Autodesk Inventor part; units mm, degrees
ref_plane "YZ Plane" through (0, 0, 0) normal (1, 0, 0) x (0, 1, 0)
ref_plane "XZ Plane" through (0, 0, 0) normal (0, 1, 0) x (-1, 0, 0)
ref_plane "XY Plane" through (0, 0, 0) normal (0, 0, 1) x (1, 0, 0)
sketch "Sketch1" plane through (0, 0, 0) normal (0, 1, 0) x (-1, 0, 0)
  line L0 (0, 0) -> (90, 0)
  line L1 (90, 0) -> (90, -52)
  line L2 (90, -60) -> (0, -60)
  line L3 (0, -60) -> (0, 0)
  line L4 (0, 0) -> (90, 0)
  line L5 (90, 0) -> (90, -8)
  line L6 (90, -8) -> (0, -8)
  line L7 (0, -8) -> (0, 0)
  line L8 (90, -60) -> (0, -60)
  line L9 (0, -60) -> (0, -52)
  line L10 (0, -52) -> (90, -52)
  line L11 (90, -52) -> (90, -60)
  line L12 (0, -8) -> (90, -8)
  line L13 (90, -8) -> (90, -12)
  line L14 (90, -12) -> (0, -12)
  line L15 (0, -12) -> (0, -8)
  line L16 (90, -52) -> (0, -52)
  line L17 (0, -52) -> (0, -48)
  line L18 (0, -48) -> (90, -48)
  line L19 (90, -48) -> (90, -52)
  line L20 (90, 0) -> (64, 0)
  line L21 (64, 0) -> (64, -8)
  line L22 (64, -8) -> (90, -8)
  line L23 (90, -8) -> (90, 0)
  line L24 (64, -8) -> (57, -8)
  line L25 (57, -8) -> (57, 0)
  line L26 (57, 0) -> (64, 0)
  line L27 (64, 0) -> (64, -8)
  line L28 (57, 0) -> (24, 0)
  line L29 (24, 0) -> (24, -8)
  line L30 (24, -8) -> (57, -8)
  line L31 (57, -8) -> (57, 0)
  line L32 (24, -8) -> (17, -8)
  line L33 (17, -8) -> (17, 0)
  line L34 (17, 0) -> (24, 0)
  line L35 (24, 0) -> (24, -8)
  line L36 (57, 0) -> (50, 0)
  line L37 (50, 0) -> (50, -8)
  line L38 (50, -8) -> (57, -8)
  line L39 (57, -8) -> (57, 0)
  line L40 (64, -52) -> (57, -52)
  line L41 (57, -52) -> (57, -60)
  line L42 (57, -60) -> (64, -60)
  line L43 (64, -60) -> (64, -52)
  line L44 (24, -52) -> (17, -52)
  line L45 (17, -52) -> (17, -60)
  line L46 (17, -60) -> (24, -60)
  line L47 (24, -60) -> (24, -52)
  dimension "d0" = 90
  dimension "d1" = 60
  dimension "d49" = 8
  dimension "d50" = 8
extrude "Extrusion1" add sketch "Sketch1" along normal blind 4 contours L14 L1 L18 L3
extrude "Extrusion2" add sketch "Sketch1" along normal blind 40 contours L0 L29 L6 L33 | L6 L1 L14 L3 | L0 L25 L6 L37 | L18 L1 L10 L3 | L0 L21 L6 L25 | L10 L47 L2 L45 | L43 L2 L41 L10
sketch "Sketch2" plane through (0, 40, 0) normal (0, 1, 0) x (1, 0, 0)
  line L0 (-64, 60) -> (-64, 52)
  line L1 (-57, 52) -> (-57, 60)
  circle A0 centre (-60.5, 55.5) radius 1.6
  line L2 (-24, 60) -> (-24, 52)
  circle A1 centre (-20.5, 56) radius 1.6
  line L3 (-90, 8) -> (-64, 8)
  circle A2 centre (-60.5, 4) radius 1.6
  line L4 (-17, 0) -> (-17, 8)
  line L5 (-24, 0) -> (-17, 0)
  circle A3 centre (-20.5, 4) radius 1.6
  point P0 (0, 0)
  point P1 (-17, 52)
  dimension "d6" = 3.2
  dimension "d7" = 3.2
  dimension "d9" = 3.2
  dimension "d10" = 3.2
extrude "Extrusion3" cut sketch "Sketch2" against normal blind 100
sketch "Sketch3" plane through (-64, 0, 0) normal (0, 0, 1) x (1, 0, 0)
  line L0 (0, 0) -> (14, 0)
  line L1 (7, 0) -> (7, 40)
  line L2 (7, 0) -> (7, 40)
  line L3 (0, 40) -> (14, 40)
  circle A0 centre (10.5, 20) radius 1
  circle A1 centre (10.5, 33) radius 1
  circle A2 centre (10.5, 7) radius 1
  point P0 (64, 0)
  dimension "d13" = 2
extrude "Extrusion4" cut sketch "Sketch3" against normal blind 30
sketch "Sketch4" plane through (0, 4, 0) normal (0, 1, 0) x (1, 0, 0)
  line L0 (0, 12) -> (-90, 12)
  line L1 (0, 48) -> (-90, 48)
  line L2 (-90, 12) -> (-86.8, 12)
  line L3 (-86.8, 12) -> (-86.8, 48)
  line L4 (-86.8, 48) -> (-90, 48)
  line L5 (-90, 48) -> (-90, 12)
  line L6 (0, 12) -> (-5, 12)
  line L7 (-5, 12) -> (-5, 48)
  line L8 (-5, 48) -> (0, 48)
  line L9 (0, 48) -> (0, 12)
  line L10 (-17, 12) -> (-10, 12)
  line L11 (-10, 12) -> (-10, 15)
  line L12 (-10, 15) -> (-17, 15)
  line L13 (-17, 15) -> (-17, 12)
  line L14 (-17, 48) -> (-10, 48)
  line L15 (-10, 48) -> (-10, 45)
  line L16 (-10, 45) -> (-17, 45)
  line L17 (-17, 45) -> (-17, 48)
  line L18 (-17, 15) -> (-10, 15)
  line L19 (-10, 21) -> (-17, 21)
  line L20 (-17, 21) -> (-10, 21)
  line L21 (-10, 21) -> (-10, 24)
  line L22 (-10, 24) -> (-17, 24)
  line L23 (-17, 24) -> (-17, 21)
  line L24 (-17, 45) -> (-10, 45)
  line L25 (-10, 39) -> (-17, 39)
  line L26 (-17, 39) -> (-10, 39)
  line L27 (-10, 39) -> (-10, 36)
  line L28 (-10, 36) -> (-17, 36)
  line L29 (-17, 36) -> (-17, 39)
  line L30 (-64, 12) -> (-71, 12)
  line L31 (-71, 12) -> (-71, 15)
  line L32 (-71, 15) -> (-64, 15)
  line L33 (-64, 15) -> (-64, 12)
  line L34 (-64, 21) -> (-71, 21)
  line L35 (-71, 21) -> (-71, 24)
  line L36 (-71, 24) -> (-64, 24)
  line L37 (-64, 24) -> (-64, 21)
  line L38 (-64, 36) -> (-71, 36)
  line L39 (-71, 36) -> (-71, 39)
  line L40 (-71, 39) -> (-64, 39)
  line L41 (-64, 39) -> (-64, 36)
  line L42 (-64, 48) -> (-71, 48)
  line L43 (-71, 48) -> (-71, 45)
  line L44 (-71, 45) -> (-64, 45)
  line L45 (-64, 45) -> (-64, 48)
  line L46 (-10, 48) -> (-17, 48)
  line L47 (-10, 12) -> (-17, 12)
  point P0 (0, 0)
  dimension "d16" = 3.2
extrude "Extrusion5" add sketch "Sketch4" along normal blind 36 contours L0 L7 L1 L9
extrude "Extrusion6" add sketch "Sketch4" along normal blind 36 contours L0 L13 L12 L11 | L15 L16 L17 L1 | L0 L31 L32 L33 | L45 L44 L43 L1
extrude "Extrusion7" add sketch "Sketch4" along normal blind 1 contours L19 L23 L22 L21 | L27 L28 L29 L25 | L34 L35 L36 L37 | L38 L39 L40 L41
sketch "Sketch5" plane through (-5, 4, -48) normal (-1, 0, 0) x (0, 0, 1)
  line L0 (0, 36) -> (36, 36)
  circle A0 centre (18, 22) radius 6
  point P0 (48, -4)
extrude "Extrusion8" cut sketch "Sketch5" against normal blind 20
sketch "Sketch6" plane through (-90, 0, -8) normal (-1, 0, 0) x (0, 0, 1)
  line L0 (0, 0) -> (-44, 0)
  line L1 (-40, 4) -> (-40, 40)
  arc A0 (-28, 12) -> (-16, 12) centre (-22, 20) ccw
  line L2 (-37, 4) -> (-37, 40)
  line L3 (-4, 12) -> (-16, 12)
  line L4 (-28, 12) -> (-37, 12)
  line L5 (-7, 4) -> (-4, 4)
  line L6 (-4, 4) -> (-4, 12)
  line L7 (-4, 40) -> (-4, 4)
  line L8 (-40, 4) -> (-4, 4)
  line L9 (-37, 12) -> (-40, 12)
  line L10 (-40, 12) -> (-40, 4)
  point P0 (8, 0)
  dimension "d30" = 20
extrude "Extrusion9" add sketch "Sketch6" against normal blind 4
sketch "Sketch8" plane through (0, 0, 0) normal (0, -1, 0) x (1, 0, 0)
  line L0 (-64, -52) -> (-90, -52)
  line L1 (-86, -52) -> (-76, -52)
  line L2 (-76, -52) -> (-76, -56)
  line L3 (-76, -56) -> (-86, -56)
  line L4 (-86, -56) -> (-86, -52)
  line L5 (-85, -52) -> (-77, -52)
  line L6 (-77, -52) -> (-77, -55)
  line L7 (-77, -55) -> (-85, -55)
  line L8 (-85, -55) -> (-85, -52)
  line L9 (-85, -55) -> (-77, -55)
  line L10 (-77, -55) -> (-77, -46.5727)
  line L11 (-77, -46.5727) -> (-85, -46.5727)
  line L12 (-85, -46.5727) -> (-85, -55)
  point P0 (0, 0)
extrude "Extrusion14" add sketch "Sketch8" against normal blind 15 contours L2 L3 L4 L0 L8 L7 L6 | L6 L7 L8 L0
extrude "Extrusion15" cut sketch "Sketch8" against normal blind 15 contours L6 L7 L8 L0 | L0 L12 L11 L10
sketch "Sketch9" plane through (0, 0, -52) normal (0, 0, -1) x (-1, 0, 0)
  line L0 (0, 0) -> (0, 40)
  line L1 (0, 0) -> (36, 0)
  line L2 (36, 0) -> (36, 11.5)
  line L3 (36, 11.5) -> (0, 11.5)
  line L4 (0, 11.5) -> (0, 0)
  circle A0 centre (36, 11.5) radius 1
  dimension "d45" = 11.5
  dimension "d46" = 2
extrude "Extrusion16" cut sketch "Sketch9" against normal blind 10 contours A0 L2 L3 | L3 L2 A0
sketch "Sketch10" plane through (-90, 0, -8) normal (-1, 0, 0) x (0, 0, 1)
  line L0 (-44, 0) -> (-52, 0)
  line L1 (-44, 0) -> (-44, 7)
  line L2 (-44, 0) -> (-44, 40)
  circle A0 centre (-33, 7) radius 1.2
  line L3 (0, 0) -> (0, 40)
  line L4 (0, 7) -> (11, 7) construction
  circle A1 centre (-11, 7) radius 1.2
  point P0 (8, 0)
  dimension "d51" = 2.4
  dimension "d54" = 2.4
properties part number "_3DPrint"
The listing builds one solid part. Answer for the finished solid, in the listing's coordinates (mm). A direction names the side the tool comes from. Coordinates: 2 decimals unless noted, no trailing zeros. Write each loop counter-clockwise with the first axis right and the second up, starting at its lowest first coordinate (ties: lowest second). Pieces come first, ordered by that corner, then holes. Notation, with made-up numbers: (29, -18.5) - (83, -18.5) arc R25 cw to (83, 5.5) - close; hole circle Ø2 at (38.5, 41). An arc over 180 degrees is marked (long way). Return JSON: item names as keys, results as strings. Group by question number.
1. Given pin 1 (1.5 mm diameter, centred on y = 31.5, z = -41, fed in from -X); pin 2 (1.5 mm diameter, centred on x = -40.5, y = 19.5, fed in from +Z); pin 3 (2 mm diameter, centred on y = 21.5, z = -27, fed in from +X); pin 4 (3 mm diameter, centred on x = -83, y = 11, fed in from -Z), each flat-ended and moving along its own axis, determine where each tip first touches the part or whether it passes through.
2. A cutting plane is placed at C-C, the plane x = -53.5. Determine the outline of the cut face in (y, z).
3. A cutting plane is placed at D-D, the plane z = -22.5. Determine the outline of the cut face in (x, y), plus the area to 3 significant figures.
4. Determine the mould class of faces 1 (the flat face through (-77, 20, -8)), 2 (the flat face through (-90, 11, -35)), 3 (the flat face through (-68, 5, -38)), 4 (the flat face through (-81, 2, -46.573)) for opening direction X: released by +X, released by -X, zero draft, split by the parting line, or undercut.
5. Straight lines are drawn through the part: L1, parallel to Z at x = -20.5, y = 13.5; L2, parallel to Z at x = -60.5, y = 8.5; L3, parallel to Z at x = -57.5, y = 34.5. For each, find the intervals that lie inside material, in ascending order.
6. A cutting plane is placed at A-A, the plane x = -36. Determine the outline of the cut face in (y, z).
7. Which of the six approach directions +Z, -Z, +X, -X, +Y, -Y give full straight-line access (tool end or side, diameter ignored) to faces 5 (the cylindrical face through (-36.954, 11.8, -50.028)), 6 (the flat face through (-81, 7, -55)), 7 (the flat face through (-88, 12, -42)), 8 (the flat face through (-77, 7, -52)), 9 (the flat face through (-68, 22, -45))?
8. A cutting plane is placed at B-B, the plane z = -30. Determine the outline of the cut face in (x, y).
Ans:
{
 "1": {"pin 1": "x = -5", "pin 2": "z = -8", "pin 3": "x = 0", "pin 4": "z = -56"},
 "2": {"outline": "(0, -52) - (40, -52) - (40, -48) - (4, -48) - (4, -12) - (6, -12) - (6, 0) - (0, 0) - close; (8, -12) - (19, -12) - (19, 0) - (8, 0) - close; (21, -12) - (32, -12) - (32, 0) - (21, 0) - close; (34, -12) - (40, -12) - (40, 0) - (34, 0) - close"},
 "3": {"outline": "(-90, 0) - (0, 0) - (0, 40) - (-5, 40) - (-5, 4) - (-10, 4) - (-10, 5) - (-17, 5) - (-17, 4) - (-64, 4) - (-64, 5) - (-71, 5) - (-71, 4) - (-86, 4) - (-86, 12) - (-90, 12) - close", "area": "586 mm²"},
 "4": {"face 1": "zero draft", "face 2": "released by -X", "face 3": "undercut", "face 4": "undercut"},
 "5": {"L1": "-60 to -57.6, -54.4 to -48, -12 to -5.6, -2.4 to 0", "L2": "-60 to -57.1, -53.9 to -48, -12 to -5.6, -2.4 to 0", "L3": "-60 to -48, -12 to 0"},
 "6": {"outline": "(0, -52) - (10.5, -52) - (10.5, -48) - (4, -48) - (4, -12) - (40, -12) - (40, -8) - (0, -8) - close; (12.5, -52) - (40, -52) - (40, -48) - (12.5, -48) - close"},
 "7": {"face 5": "-Z", "face 6": "+Y, -Y", "face 7": "-X, +Y", "face 8": "-Y", "face 9": "+Y"},
 "8": {"outline": "(-90, 0) - (0, 0) - (0, 20) - (-5, 20) - (-5, 4) - (-86, 4) - (-86, 10) - (-90, 10) - close; (-5, 32) - (0, 32) - (0, 40) - (-5, 40) - close"}
}
